```python
from build123d import *

# Parameters (mm, degrees)
SKETCH1_R                    = 36.5125
BOSS_EXTRUDE1_DEPTH          = 12.7
F_1_4_20_TAPPED_HOLE1_D      = 5.1054
F_3_8_0_375_DIAMETER_HOLE1_D = 10.3124
CIRPATTERN1_COUNT            = 8


with BuildPart() as part:
    # Sketch1 → Boss-Extrude1 (new body)
    with BuildSketch(Plane.XY):
        Circle(SKETCH1_R)
    extrude(amount=BOSS_EXTRUDE1_DEPTH)

    # 1_4-20 Tapped Hole1 (through all)
    with Locations(Plane.XY.offset(12.7)):
        with Locations((9.525, 0), (-9.525, 0)):
            Hole(F_1_4_20_TAPPED_HOLE1_D / 2)

    # 3_8 _0.375_ Diameter Hole1 (through all)
    with Locations(Plane.XY.offset(12.7)):
        with Locations((25.4, 0)):
            f_3_8_0_375_diameter_hole1 = Hole(F_3_8_0_375_DIAMETER_HOLE1_D / 2)

    # CirPattern1: 3_8 _0.375_ Diameter Hole1 ×8 about axis
    cirpattern1_axis = Axis((0, 0, 0), (0, 0, 1))
    for i in range(1, CIRPATTERN1_COUNT):
        add(f_3_8_0_375_diameter_hole1.rotate(cirpattern1_axis, i * 360 / CIRPATTERN1_COUNT), mode=Mode.SUBTRACT)


solid = part.part
```
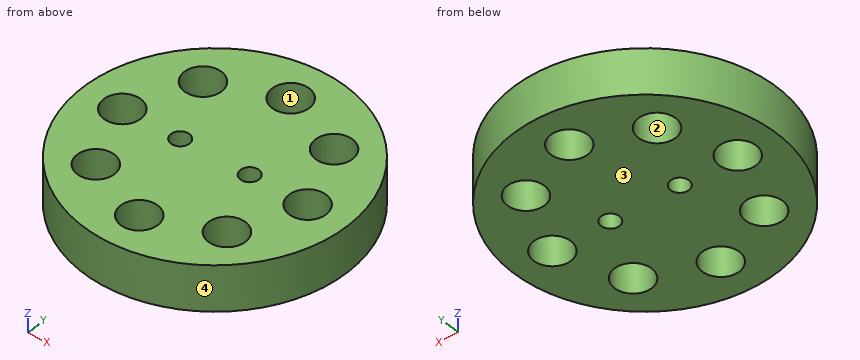
Geometry check sheet. Reference: the model listing, model coordinates, mm. Face numbers are marked on the shaded views. Round coordinates to 2 decimals unless told otherwise and drop trailing zeros. Loops run counter-clockwise (first coordinate to the right, second up) from the corner with the lowest first, then second, coordinate; pieces in that order, holes last. Notation, with made-up numbers: (0, 3) - (5, 3) arc R21 ccw to (5, 26) - close; hole circle Ø3 at (-25, -18.75). An arc over 180 degrees is marked (long way). Write item = value, one per line. Start each with the question number.
1. Section check B-B on y = -25.4. Enter the section's corners in (x, z).
2. Thickness scan on line 1 (X direction, y = -2, z = 1.5); line 2 (Y direction, x = -0.5, z = 9); line 3 (Y direction, x = 17, z = 3). Record the ranges inside material, lowest first.
3. Depth check by flat-ended pin: pin 1 (8 mm diameter, centred on x = -17.96, y = -17.96, fed in from +Z); pin 2 (6 mm diameter, centred on x = 20.5, z = 8.5, fed in from +Y); pin 3 (5 mm diameter, centred on y = 24, z = 10, fed in from +X); pin 4 (5 mm diameter, centred on x = -9, z = 6, fed in from +Y). Enter the tip coordinate at first touch or a pass-through.
4. Mould release check, pull along Y, two halves, no side actions. Record for the marked faces 1, 2, 3 and 4: released by +Y, released by -Y, zero draft, split by the parting line, or undercut.
5. Section check A-A on x = 0. Enter the section's corners in (y, z).
6. Section check D-D on z = 8. Give the number of separate pieces and of enclosed holes in the cut face, then the cut area to 3 significant figures.
Working result:
q1.outline = (-26.23, 0) - (-5.16, 0) - (-5.16, 12.7) - (-26.23, 12.7) - close; (5.16, 0) - (26.23, 0) - (26.23, 12.7) - (5.16, 12.7) - close
q2.line_1 = -36.46 to -30.15, -20.65 to -11.11, -7.94 to 7.94, 11.11 to 20.65, 30.15 to 36.46
q2.line_2 = -36.51 to -30.53, -20.27 to 20.27, 30.53 to 36.51
q2.line_3 = -32.31 to -23.03, -12.89 to 12.89, 23.03 to 32.31
q3.pin_1 = through
q3.pin_2 = 32.05
q3.pin_3 = 29.51
q3.pin_4 = 35.93
q4.face_1 = undercut
q4.face_2 = undercut
q4.face_3 = zero draft
q4.face_4 = split by the parting line
q5.outline = (-36.51, 0) - (-30.56, 0) - (-30.56, 12.7) - (-36.51, 12.7) - close; (-20.24, 0) - (20.24, 0) - (20.24, 12.7) - (-20.24, 12.7) - close; (30.56, 0) - (36.51, 0) - (36.51, 12.7) - (30.56, 12.7) - close
q6.separate_pieces = 1
q6.enclosed_holes = 10
q6.area = 3,480 mm^2
